For this review, take the finished solid that the model builds, in its own axes (mm). Face numbers are marked on the shaded views. Coordinates: 2 decimals unless noted, no trailing zeros. Loops run counter-clockwise (first coordinate to the right, second up) from the corner with the lowest first, then second, coordinate; pieces in that order, holes last. Notation, with made-up numbers: (-16.75, -5) - (6.25, -5) arc R26 ccw to (6.25, 29) - close; hole circle Ø1 at (-14.5, 28.5). An arc over 180 degrees is marked (long way). Answer as a JSON object with one key per item and string values. Group by question number.
Item 1: To check wall thickness, follow line 1 (Z direction, x = 1.5, y = 0.2); line 2 (X direction, y = 1.45, z = 4.5); line 3 (X direction, y = 0.2, z = 28.5). State the ranges of each line that lie inside material, in increasing order.
Item 2: Clearance check with a flat-ended pin moving along its axis: pin 1 (1.5 mm diameter, centred on x = -10, z = -1.5, fed in from +Y). State where the tip first meets the part, or that it passes through.
Item 3: We need section A-A (z = 3.5). Give the boundary of the cut face in (x, y).
Item 4: We need section B-B (x = 0). Give the boundary of the cut face in (y, z), then the cut area to 3 significant figures.
Item 5: We need section D-D (z = 19). Give the boundary of the cut face in (x, y).
Item 6: We need section C-C (x = 5.25). Give the boundary of the cut face in (y, z).
Item 7: Mouldability with a two-part tool opening along Z and no side actions: class the marked faces 1 and 2 as released by +Z, released by -Z, zero draft, split by the parting line, or undercut.
from build123d import *

# Parameters (mm, degrees)
SKETCH3_W           = 29
SKETCH3_H           = 46.502559765
SKETCH3_R           = 2.6
BOSS_EXTRUDE1_DEPTH = 3
SKETCH4_W           = 20.4
SKETCH4_H           = 20.4
CUT_EXTRUDE1_DEPTH  = 1
CUT_EXTRUDE2_DEPTH  = 1.5
SKETCH6_R           = 1.025
CUT_EXTRUDE3_DEPTH  = 1.5
CUT_EXTRUDE4_DEPTH  = 1.5


with BuildPart() as part:
    # Sketch3 → Boss-Extrude1 (new body)
    with BuildSketch(Plane(origin=(0, 0, 0), x_dir=(1, 0, 0), z_dir=(0, 1, 0))):
        with Locations((-0.002492114, -8.748720117)):
            Rectangle(SKETCH3_W, SKETCH3_H)
        with Locations((0, -19)):
            Circle(SKETCH3_R, mode=Mode.SUBTRACT)
    extrude(amount=BOSS_EXTRUDE1_DEPTH)

    # Sketch4 → Cut-Extrude1 (cut)
    with BuildSketch(Plane.XZ):
        with Locations((0, 19)):
            Rectangle(SKETCH4_W, SKETCH4_H)
    extrude(amount=-CUT_EXTRUDE1_DEPTH, mode=Mode.SUBTRACT)

    # Sketch5 → Cut-Extrude2 (cut)
    with BuildSketch(Plane(origin=(0, 3, 0), x_dir=(1, 0, 0), z_dir=(0, 1, 0))):
        with BuildLine():
            Line((-12.00249203, 8.502556434), (-12.00249175, -8.502983271))
            ThreePointArc((-12.00249175, -8.502983271), (-10.973497147, -10.976182335), (-8.497093239, -11.997440002))
            Line((-8.497093239, -11.997440002), (8.497508549, -11.997440458))
            ThreePointArc((8.497508549, -11.997440458), (10.972380637, -10.972314999), (11.99750783, -8.497443607))
            Line((11.99750783, -8.497443607), (11.997507522, 8.497016765))
            ThreePointArc((11.997507522, 8.497016765), (10.976250085, 10.973564476), (8.502907209, 12.002559308))
            Line((8.502907209, 12.002559308), (4.502491803, 12.00255968))
            Line((4.502491803, 12.00255968), (4.502491803, 14.502559765))
            Line((4.502491803, 14.502559765), (-4.502491803, 14.502559765))
            Line((-4.502491803, 14.502559765), (-4.502491803, 12.002559739))
            Line((-4.502491803, 12.002559739), (-8.502491889, 12.002559765))
            ThreePointArc((-8.502491889, 12.002559765), (-10.977366841, 10.977432329), (-12.00249203, 8.502556434))
        make_face()
    extrude(amount=-CUT_EXTRUDE2_DEPTH, mode=Mode.SUBTRACT)

    # Sketch6 → Cut-Extrude3 (cut)
    with BuildSketch(Plane(origin=(0, 1.5, 0), x_dir=(1, 0, 0), z_dir=(0, 1, 0))):
        with Locations((-8.502491891, 8.502559653)):
            Circle(SKETCH6_R)
        with Locations((8.497508109, 8.502559653)):
            Circle(SKETCH6_R)
        with Locations((8.497507663, -8.497440347)):
            Circle(SKETCH6_R)
        with Locations((-8.502492337, -8.497440347)):
            Circle(SKETCH6_R)
    extrude(amount=-CUT_EXTRUDE3_DEPTH, mode=Mode.SUBTRACT)

    # Sketch7 → Cut-Extrude4 (cut)
    with BuildSketch(Plane(origin=(0, 1.5, 0), x_dir=(1, 0, 0), z_dir=(0, 1, 0))):
        with BuildLine():
            Line((-6.002491891, 8.502559653), (5.997508109, 8.502559653))
            ThreePointArc((5.997508109, 8.502559653), (6.729741157, 6.7347927), (8.497508109, 6.002559653))
            Line((8.497508109, 6.002559653), (8.497508109, -5.997440347))
            ThreePointArc((8.497508109, -5.997440347), (6.729740868, -6.729673236), (5.997507663, -8.497440347))
            Line((5.997507663, -8.497440347), (-6.002492337, -8.497440347))
            ThreePointArc((-6.002492337, -8.497440347), (-6.734725226, -6.729673552), (-8.502491891, -5.997440347))
            Line((-8.502491891, -5.997440347), (-8.502491891, 6.002559653))
            ThreePointArc((-8.502491891, 6.002559653), (-6.734724938, 6.7347927), (-6.002491891, 8.502559653))
        make_face()
    extrude(amount=-CUT_EXTRUDE4_DEPTH, mode=Mode.SUBTRACT)


solid = part.part
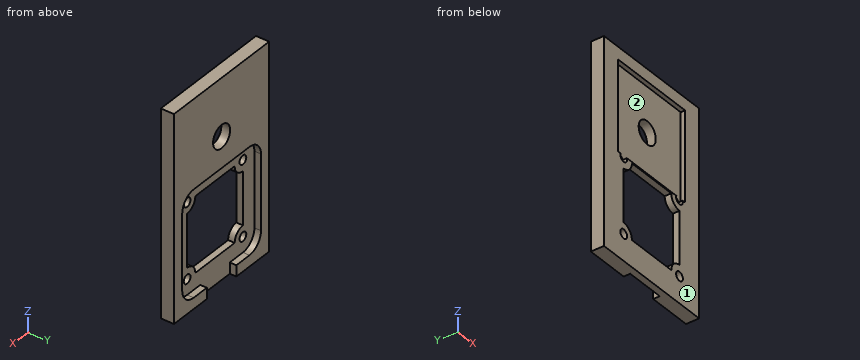
Check sheet entries:
{
 "1": {"line 1": "z = -14.5 to -8.5, 8.5 to 8.8, 29.2 to 32", "line 2": "x = -14.5 to -8.5, 8.5 to 14.5", "line 3": "x = -14.5 to -10.2, 10.2 to 14.5"},
 "2": {"pin 1": "stops at y = 1.5"},
 "3": {"outline": "(-14.5, 0) - (-8.5, 0) - (-8.5, 1.5) - (-12, 1.5) - (-12, 3) - (-14.5, 3) - close; (8.5, 0) - (14.5, 0) - (14.5, 3) - (12, 3) - (12, 1.5) - (8.5, 1.5) - close"},
 "4": {"outline": "(0, -14.5) - (1.5, -14.5) - (1.5, -8.5) - (0, -8.5) - close; (0, 8.5) - (1.5, 8.5) - (1.5, 12) - (3, 12) - (3, 16.4) - (1, 16.4) - (1, 8.8) - (0, 8.8) - close; (0, 29.2) - (1, 29.2) - (1, 21.6) - (3, 21.6) - (3, 32) - (0, 32) - close", "area": "43.5 mm2"},
 "5": {"outline": "(-14.5, 0) - (-10.2, 0) - (-10.2, 1) - (-2.6, 1) - (-2.6, 3) - (-14.5, 3) - close; (2.6, 1) - (10.2, 1) - (10.2, 0) - (14.5, 0) - (14.5, 3) - (2.6, 3) - close"},
 "6": {"outline": "(0, -14.5) - (3, -14.5) - (3, -12) - (1.5, -12) - (1.5, -8.5) - (0, -8.5) - close; (0, 8.5) - (1.5, 8.5) - (1.5, 12) - (3, 12) - (3, 32) - (0, 32) - (0, 29.2) - (1, 29.2) - (1, 8.8) - (0, 8.8) - close"},
 "7": {"face 1": "zero draft", "face 2": "undercut"}
}
